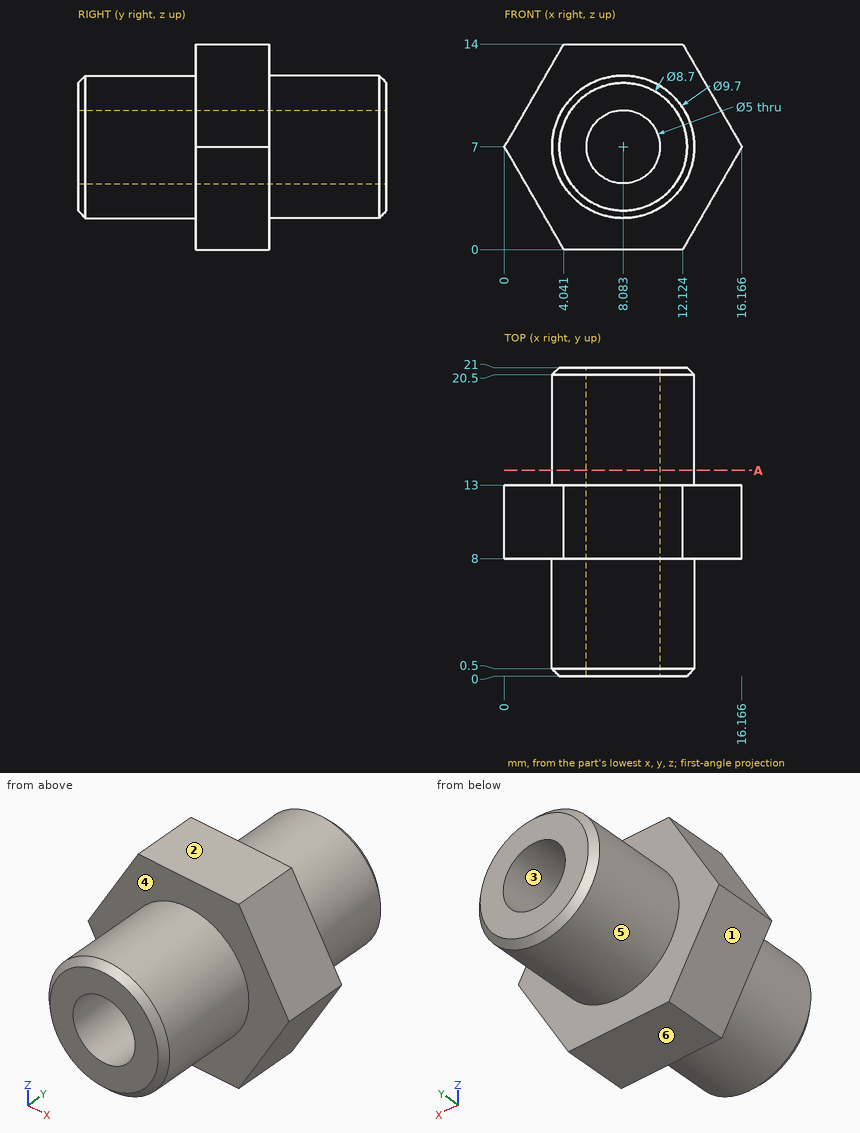
For this review, use the dimensioned drawing (mm, ordinates from the lowest corner) and the shaded views. A direction names the side the tool comes from. Coordinates: 2 decimals unless noted, no trailing zeros. Write each loop counter-clockwise with the first axis right and the second up, starting at its lowest first coordinate (ties: lowest second). Pieces come first, ordered by that corner, then holes. Notation, with made-up numbers: (-38, 8.5) - (-32, 8.5) arc R21 cw to (-32, 44.5) - close; hole circle Ø9 at (73.25, 55). An arc over 180 degrees is marked (long way). Answer as a JSON object with one key per item and string values. Group by question number.
1. To check wall thickness, follow probe 1 along Y at (x, z) = (13.25, 2.75); probe 2 along X at (y, z) = (14.5, 7); probe 3 along Z at (x, y) = (8, 5.5). State the ranges of each line that lie inside material, in increasing order.
2. Add section A-A (y = 14). Give the boundary of the cut face in (x, z).
3. Mouldability with a two-part tool opening along Z and no side actions: class the marked faces 1, 2 and 3 as pulls with the +Z half, pulls with the -Z half, needs draft (parallel to the pull), parting line crosses it, or undercut.
4. Clearance check with a flat-ended pin moving along its axis: pin 1 Ø1.5 at (y, z) = (15, 11.5) entering from -X. State where the tip first meets the part, or that it passes through.
5. Machinability: for the marked faces 4, 5 and 6, which of the approach directions +Z, -Z, +X, -X, +Y, -Y give a long, thin tool a straight path to every point of the face, cutting with its end or side? Answer none if there is none.
Findings:
{
 "1": {"probe 1": "8 to 13", "probe 2": "3.23 to 5.58, 10.58 to 12.93", "probe 3": "2.15 to 4.5, 9.5 to 11.85"},
 "2": {"outline": "circle Ø9.7 at (8.08, 7); hole circle Ø5 at (8.08, 7)"},
 "3": {"face 1": "pulls with the -Z half", "face 2": "pulls with the +Z half", "face 3": "undercut"},
 "4": {"pin 1": "x = 5.01"},
 "5": {"face 4": "-Y", "face 5": "+Y", "face 6": "-Z, +X, -X, +Y, -Y"}
}
